Work out the finished part from the listing and answer in its coordinate system (mm). Face numbers are marked on the shaded views. Coordinates: 2 decimals unless noted, no trailing zeros. Write each loop counter-clockwise with the first axis right and the second up, starting at its lowest first coordinate (ties: lowest second). Pieces come first, ordered by that corner, then holes. Notation, with made-up numbers: (-12.5, -19) -> (-7.5, -19) arc R20 cw to (-7.5, -12) -> close; hole circle Ø10 at (30.5, -5). An arc over 180 degrees is marked (long way). Write each question's results on one line, items separated by ' | '. Start each with the question number.
from build123d import *

# Parameters (mm, degrees)
F0_R     = 18.5
F2_R     = 20
F4_T     = 4
F5_R     = 18.5
F6_DEPTH = 25


with BuildPart() as f3:
    # F0 (on Top) → F3 section 0
    with BuildSketch(Plane.XY):
        Circle(F0_R)
    # F2 (on offset) → F3 section 1
    with BuildSketch(Plane.XY.offset(15)):
        Circle(F2_R)
    loft()

    # F4
    f4_openings = [f3.faces().sort_by_distance(p)[0] for p in [
        (0, 0, 15),
    ]]
    offset(amount=F4_T, openings=f4_openings, kind=Kind.INTERSECTION)

    # F5 (on face) → F6 (cut)
    with BuildSketch(Plane.XY):
        Circle(F5_R)
    extrude(amount=-F6_DEPTH, mode=Mode.SUBTRACT)


solid = f3.part
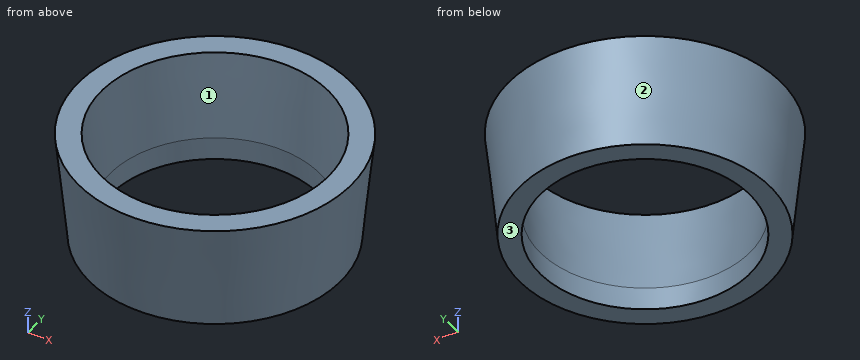
1. Given pin 1 Ø8 at (y, z) = (-4.5, -2) entering from -X; pin 2 Ø10 at (y, z) = (-2, 3) entering from +X; pin 3 Ø3 at (x, z) = (-4.5, 9.5) entering from +Y, each flat-ended and moving along its own axis, determine where each tip first touches the part or whether it passes through.
2. Find section C-C on z = 8. Give the vertices of the cut face in (x, y), and give its area (3 significant figures).
3. Find the intervals of material crossed by L1, parallel to Y at x = -8, z = 4.5; L2, parallel to Y at x = 11.5, z = -0.25; L3, parallel to X at y = -7, z = 11.75, in increasing order.
4. Find section B-B on z = 3.75. Give the vertices of the cut face in (x, y) (3 decimals), and give its area (3 significant figures).
5. Determine the mould class of the marked faces 1, 2 and 3 for opening direction Y: pulls with the +Y half, pulls with the -Y half, needs draft (parallel to the pull), parting line crosses it, or undercut.
6. Find section A-A on x = 0. Give the vertices of the cut face in (y, z).
Ans:
1) pin 1: stops at x = -22.54 | pin 2: stops at x = 23.29 | pin 3: stops at y = 23.33
2) outline: circle Ø46.64 at (0, 0); hole circle Ø38.6 at (0, 0) | area: 538 mm²
3) L1: y = -21.53 to -17.18, 17.18 to 21.53 | L2: y = -19.33 to -14.49, 14.49 to 19.33 | L3: x = -22.64 to -18.39, 18.39 to 22.64
4) outline: circle Ø45.79 at (0, 0); hole circle Ø37.75 at (0, 0) | area: 528 mm²
5) face 1: undercut | face 2: parting line crosses it | face 3: needs draft
6) outline: (-24.02, 15) -> (-22.12, -4) -> (-18.5, -4) -> (-18.5, 0) -> (-20, 15) -> close; (18.5, -4) -> (22.12, -4) -> (24.02, 15) -> (20, 15) -> (18.5, 0) -> close
